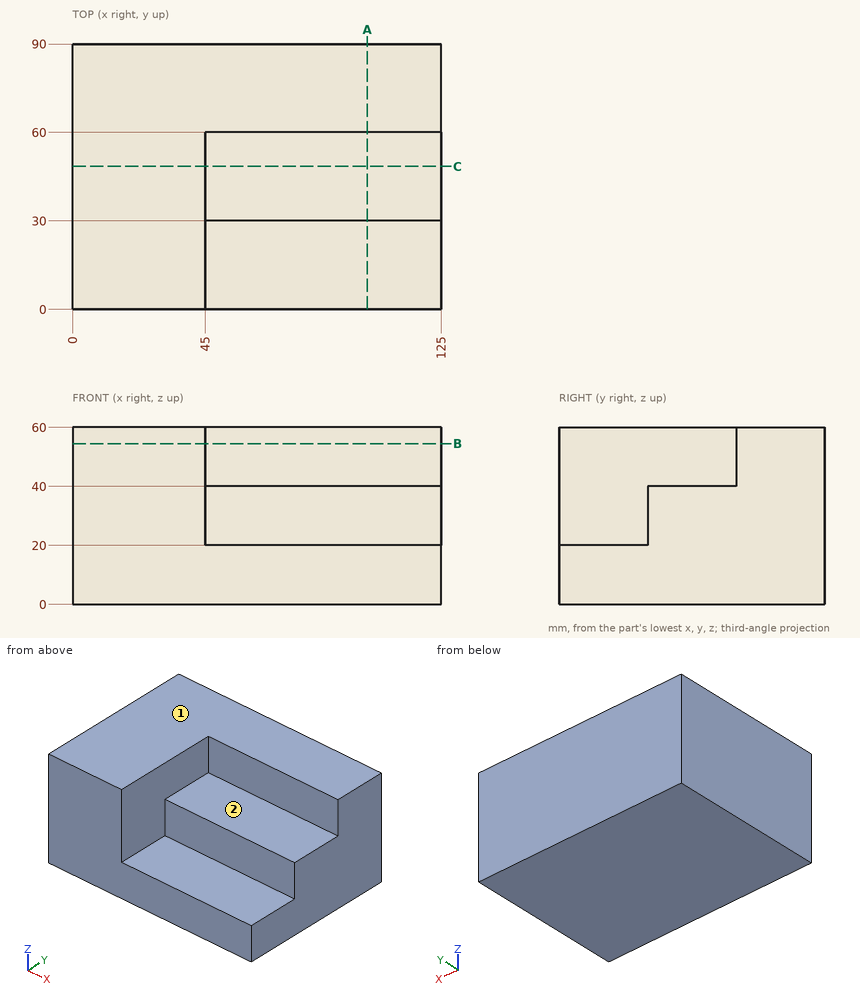
Could you check a few things on this drawing? It's one solid part, dimensions in mm from its lowest x, y, z. A direction names the side the tool comes from. Give positions to 0.01 mm unless a question says otherwise; leave off trailing zeros. Loops run counter-clockwise (first coordinate to the right, second up) from the corner with the lowest first, then second, coordinate; pieces in that order, holes last. Notation, with made-up numbers: (23.5, 35) -> (53.5, 35) arc R13 ccw to (53.5, 47) -> close; hole circle Ø10 at (30.5, 6.5). An arc over 180 degrees is marked (long way). Use one line per item in the form item = value. Start each with the question number.
1) Imagine slicing it at B-B (z = 54.5). Please give me the cut outline in (x, y).
2) Which directions (+Z, -Z, +X, -X, +Y, -Y) give clear straight access to the entire face, cutting with the end or side of a thin tool? Please do the marked faces 1 and 2.
3) Imagine slicing it at C-C (y = 48.5). Please give me the cut outline in (x, z), then the cut area to 3 significant figures.
4) Imagine slicing it at A-A (x = 100). Please give me the cut outline in (y, z), then the cut area to 3 significant figures.
5) For P1, Ø1, axis at y = 67, z = 45, coming from the -X side; P2, Ø16, axis at x = 89.5, z = 32, coming from the -Y side; P3, Ø9, axis at x = 91.5, y = 49.5, coming from the +Z side; P4, Ø9, axis at x = 89, y = 10.5, coming from the +Z side, each with a flat end and sliding along its axis, tell me the tip position at first contact or that it passes through.
6) Please list where these lines run through material, in increasing order: line 1 along Y through (x, z) = (114.5, 39); line 2 along Z through (x, y) = (63.5, 22); line 3 along Z through (x, y) = (52.5, 35.5).
Check values:
q1.outline = (0, 0) -> (45, 0) -> (45, 60) -> (125, 60) -> (125, 90) -> (0, 90) -> close
q2.face_1 = +Z, +X, -X, +Y, -Y
q2.face_2 = +Z, +X, -Y
q3.outline = (0, 0) -> (125, 0) -> (125, 40) -> (45, 40) -> (45, 60) -> (0, 60) -> close
q3.area = 5,900 mm^2
q4.outline = (0, 0) -> (90, 0) -> (90, 60) -> (60, 60) -> (60, 40) -> (30, 40) -> (30, 20) -> (0, 20) -> close
q4.area = 3,600 mm^2
q5.P1 = 0
q5.P2 = 30
q5.P3 = 40
q5.P4 = 20
q6.line_1 = 30 to 90
q6.line_2 = 0 to 20
q6.line_3 = 0 to 40
